Autodesk Inventor part; units mm, degrees
ref_plane "YZ Plane" through (0, 0, 0) normal (1, 0, 0) x (0, 1, 0)
ref_plane "XZ Plane" through (0, 0, 0) normal (0, 1, 0) x (-1, 0, 0)
ref_plane "XY Plane" through (0, 0, 0) normal (0, 0, 1) x (1, 0, 0)
sketch "Sketch1" plane through (0, 0, 0) normal (0, 1, 0) x (-1, 0, 0)
  line L0 (0, 0) -> (-296, 0)
  line L1 (-296, 0) -> (-296, -110)
  line L2 (-296, -110) -> (0, -110)
  line L3 (0, -110) -> (0, 0)
  dimension "d0" = 296
  dimension "d1" = 110
extrude "Extrusion1" add sketch "Sketch1" along normal blind 6.5
sketch "Sketch2" plane through (0, 6.5, 0) normal (0, 1, 0) x (1, 0, 0)
  line L0 (296, 0) -> (296, 110)
  line L1 (296, 110) -> (0, 110)
  line L2 (0, 110) -> (0, 0)
  line L3 (8, 110) -> (16, 110)
  line L4 (16, 110) -> (16, 114.5)
  line L5 (14, 116.5) -> (10, 116.5)
  line L6 (8, 114.5) -> (8, 110)
  line L7 (62.4, 110) -> (70.4, 110)
  line L8 (70.4, 110) -> (70.4, 114.5)
  line L9 (68.4, 116.5) -> (64.4, 116.5)
  line L10 (62.4, 114.5) -> (62.4, 110)
  line L11 (116.8, 110) -> (124.8, 110)
  line L12 (124.8, 110) -> (124.8, 114.5)
  line L13 (122.8, 116.5) -> (118.8, 116.5)
  line L14 (116.8, 114.5) -> (116.8, 110)
  line L15 (171.2, 110) -> (179.2, 110)
  line L16 (179.2, 110) -> (179.2, 114.5)
  line L17 (177.2, 116.5) -> (173.2, 116.5)
  line L18 (171.2, 114.5) -> (171.2, 110)
  line L19 (225.6, 110) -> (233.6, 110)
  line L20 (233.6, 110) -> (233.6, 114.5)
  line L21 (231.6, 116.5) -> (227.6, 116.5)
  line L22 (225.6, 114.5) -> (225.6, 110)
  line L23 (280, 110) -> (288, 110)
  line L24 (288, 110) -> (288, 114.5)
  line L25 (286, 116.5) -> (282, 116.5)
  line L26 (280, 114.5) -> (280, 110)
  arc A0 (10, 116.5) -> (8, 114.5) centre (10, 114.5) ccw
  arc A1 (16, 114.5) -> (14, 116.5) centre (14, 114.5) ccw
  arc A2 (64.4, 116.5) -> (62.4, 114.5) centre (64.4, 114.5) ccw
  arc A3 (70.4, 114.5) -> (68.4, 116.5) centre (68.4, 114.5) ccw
  arc A4 (118.8, 116.5) -> (116.8, 114.5) centre (118.8, 114.5) ccw
  arc A5 (124.8, 114.5) -> (122.8, 116.5) centre (122.8, 114.5) ccw
  arc A6 (173.2, 116.5) -> (171.2, 114.5) centre (173.2, 114.5) ccw
  arc A7 (179.2, 114.5) -> (177.2, 116.5) centre (177.2, 114.5) ccw
  arc A8 (227.6, 116.5) -> (225.6, 114.5) centre (227.6, 114.5) ccw
  arc A9 (233.6, 114.5) -> (231.6, 116.5) centre (231.6, 114.5) ccw
  arc A10 (282, 116.5) -> (280, 114.5) centre (282, 114.5) ccw
  arc A11 (288, 114.5) -> (286, 116.5) centre (286, 114.5) ccw
  line L27 (16, 112.25) -> (62.4, 112.25) construction
  line L28 (70.4, 112.25) -> (116.8, 112.25) construction
  line L29 (124.8, 112.25) -> (171.2, 112.25) construction
  line L30 (179.2, 112.25) -> (225.6, 112.25) construction
  line L31 (233.6, 112.25) -> (280, 112.25) construction
  line L32 (0, 55) -> (296, 55) construction
  line L33 (0, 0) -> (296, 0)
  line L34 (296, 0) -> (296, 110)
  line L35 (296, 110) -> (0, 110)
  line L36 (0, 110) -> (0, 0)
  line L37 (8, 0) -> (16, 0)
  line L38 (16, 0) -> (16, -7.5)
  line L39 (14, -9.5) -> (10, -9.5)
  line L40 (8, -7.5) -> (8, 0)
  line L41 (62.4, 0) -> (70.4, 0)
  line L42 (70.4, 0) -> (70.4, -7.5)
  line L43 (68.4, -9.5) -> (64.4, -9.5)
  line L44 (62.4, -7.5) -> (62.4, 0)
  line L45 (116.8, 0) -> (124.8, 0)
  line L46 (124.8, 0) -> (124.8, -7.5)
  line L47 (122.8, -9.5) -> (118.8, -9.5)
  line L48 (116.8, -7.5) -> (116.8, 0)
  line L49 (171.2, 0) -> (179.2, 0)
  line L50 (179.2, 0) -> (179.2, -7.5)
  line L51 (177.2, -9.5) -> (173.2, -9.5)
  line L52 (171.2, -7.5) -> (171.2, 0)
  line L53 (225.6, 0) -> (233.6, 0)
  line L54 (233.6, 0) -> (233.6, -7.5)
  line L55 (231.6, -9.5) -> (227.6, -9.5)
  line L56 (225.6, -7.5) -> (225.6, 0)
  line L57 (280, 0) -> (288, 0)
  line L58 (288, 0) -> (288, -7.5)
  line L59 (286, -9.5) -> (282, -9.5)
  line L60 (280, -7.5) -> (280, 0)
  arc A12 (8, -7.5) -> (10, -9.5) centre (10, -7.5) ccw
  arc A13 (14, -9.5) -> (16, -7.5) centre (14, -7.5) ccw
  arc A14 (62.4, -7.5) -> (64.4, -9.5) centre (64.4, -7.5) ccw
  arc A15 (68.4, -9.5) -> (70.4, -7.5) centre (68.4, -7.5) ccw
  arc A16 (116.8, -7.5) -> (118.8, -9.5) centre (118.8, -7.5) ccw
  arc A17 (122.8, -9.5) -> (124.8, -7.5) centre (122.8, -7.5) ccw
  arc A18 (171.2, -7.5) -> (173.2, -9.5) centre (173.2, -7.5) ccw
  arc A19 (177.2, -9.5) -> (179.2, -7.5) centre (177.2, -7.5) ccw
  arc A20 (225.6, -7.5) -> (227.6, -9.5) centre (227.6, -7.5) ccw
  arc A21 (231.6, -9.5) -> (233.6, -7.5) centre (231.6, -7.5) ccw
  arc A22 (280, -7.5) -> (282, -9.5) centre (282, -7.5) ccw
  arc A23 (286, -9.5) -> (288, -7.5) centre (286, -7.5) ccw
  dimension "d4" = 2
  dimension "d5" = 8
  dimension "d6" = 8
  dimension "d7" = 8
  dimension "d8" = 8
  dimension "d9" = 8
  dimension "d10" = 8
  dimension "d11" = 6.5
  dimension "d12" = 8
  dimension "d13" = 8
  dimension "d16" = 2
  dimension "d17" = 9.5
extrude "Extrusion3" add sketch "Sketch2" against normal blind 6.5 contours L58 A23 L59 A22 L60 L33 | L1 L26 A10 L25 A11 L24 | L54 A21 L55 A20 L56 L33 | L1 L22 A8 L21 A9 L20 | L50 A19 L51 A18 L52 L33 | L1 L18 A6 L17 A7 L16 | L46 A17 L47 A16 L48 L33 | L1 L14 A4 L13 A5 L12 | L42 A15 L43 A14 L44 L33 | L1 L10 A2 L9 A3 L8 | L38 A13 L39 A12 L40 L33 | L1 L6 A0 L5 A1 L4
equation "\"d6\" = d5"
equation "\"d7\" = d6"
equation "\"d8\" = d7"
equation "\"d9\" = d8"
equation "\"d10\" = d9"
equation "\"d13\" = d12"
properties part number "spool_stand_brace_bottom" material "Plywood, Finish"
Can you work these out from the model? Positions are in its coordinate system, mm. A direction names the side the tool comes from. Round coordinates to 2 decimals unless told otherwise and drop trailing zeros. Write each loop counter-clockwise with the first axis right and the second up, starting at its lowest first coordinate (ties: lowest second). Pieces come first, ordered by that corner, then holes. Notation, with made-up numbers: (45.25, 36) -> (99.25, 36) arc R12 ccw to (99.25, 51) -> close; hole circle Ø9 at (40.5, 69.25). An arc over 180 degrees is marked (long way). One line per question, with ' | ' between items. Start each with the question number.
1) On a 3-axis mill with a long thin cutter (end or side, diameter ignored), from which of +Z, -Z, +X, -X, +Y, -Y can I reach the whole of each face in a straight line? I mean faces 1 (the flat face through (292, 3, 0)), 2 (the flat face through (257, 3, -110)), 3 (the flat face through (233.6, 3, 4)). Say none if no direction works.
2) If we mould it in two halves opening along X, with no side actions, what happens to faces 4 (the flat face through (256, 3, 0)), 5 (the flat face through (288, 3, 4)), 6 (the flat face through (8, 3, 4))? For each: released by +X, released by -X, zero draft, split by the parting line, or undercut.
3) I need wall thicknesses on line 1 (X direction, y = 2.25, z = 3); line 2 (Z direction, x = 51, y = 2); line 3 (Z direction, x = 227, y = 2.25). Which ranges of each line are inside material? Lowest first, please. Write a range as [from, to].
4) Suppose I cut it at A-A on x = 241.5. Write out the boundary of the cut face in (y, z).
5) I'm going to push flat-ended pins straight in: P1, Ø1.3, axis at y = 4, z = -112.5, coming from the +X side; P2, Ø3, axis at x = 49, y = 2, coming from the -Z side; P3, Ø3, axis at x = 83, y = 2, coming from the +Z side. Where does each tip first touch, or does it pass through?
Return value:
1) face 1: +Z, +X, +Y, -Y | face 2: -Z, +Y, -Y | face 3: +Z, +Y, -Y
2) face 4: undercut | face 5: released by +X | face 6: released by -X
3) line 1: x = [8, 16], [62.4, 70.4], [116.8, 124.8], [171.2, 179.2], [225.6, 233.6], [280, 288] | line 2: z = [-110, 0] | line 3: z = [-116.41, 9.41]
4) outline: (0, -110) -> (6.5, -110) -> (6.5, 0) -> (0, 0) -> close
5) P1: stops at x = 288 | P2: stops at z = -110 | P3: stops at z = 0
